Autodesk Inventor part; units mm, degrees
ref_plane "ANBAU_XY" through (0, 5.2, 8.6) normal (0, 0, -1) x (1, 0, 0)
ref_plane "ANBAU_YZ" through (0, 5.2, 8.6) normal (1, 0, 0) x (0, -1, 0)
ref_plane "ANBAU_ZX" through (0, 5.2, 8.6) normal (0, -1, 0) x (0, 0, -1)
sketch "Skizze_1" plane through (0, 0, 0) normal (0, 0, 1) x (1, 0, 0)
  line L0 (-6, 20.5) -> (-6, 0)
  line L1 (-6, 0) -> (6, 0)
  line L2 (6, 0) -> (6, 20.5)
  arc A0 (6, 20.5) -> (2, 24.5) centre (2, 20.5) ccw
  line L3 (2, 24.5) -> (-2, 24.5)
  arc A1 (-2, 24.5) -> (-6, 20.5) centre (-2, 20.5) ccw
extrude "Extrusion1" add sketch "Skizze_1" along normal blind 19
sketch "Skizze_2" plane through (0, 0, 0) normal (1, 0, 0) x (0, 1, 0)
  line L0 (1.5, 8.6) -> (0, 8.6)
  line L1 (0, 8.6) -> (0, 7.734)
  line L2 (0, 7.734) -> (1.5, 8.6)
extrude "Extrusion2" cut sketch "Skizze_2" along normal mid plane 12
sketch "Skizze_5" plane through (0, 0, 0) normal (1, 0, 0) x (0, 1, 0)
  line L0 (5.2, 0) -> (5.2, 8.6)
  line L1 (5.2, 0.6) -> (8.3, 0.6)
  line L2 (8.3, 0.6) -> (8.7, 1)
  line L3 (8.7, 1) -> (8.7, 4.6)
  line L4 (8.7, 4.6) -> (9.2, 4.6)
  line L5 (9.2, 4.6) -> (9.2, 0)
  line L6 (9.2, 0) -> (5.2, 0)
  line L7 (5.2, 0) -> (5.2, 0.6)
sketch "Sketch_1" plane through (0, 0, 8.6) normal (0, 0, 1) x (1, 0, 0)
  line L0 (-6, 24.5) -> (-6, 0)
  line L1 (-6, 0) -> (8, 0)
  line L2 (8, 0) -> (8, 15)
  line L3 (8, 15) -> (6, 15)
  arc A0 (2, 11) -> (6, 15) centre (2, 15) ccw
  line L4 (2, 11) -> (-2.8, 11)
  line L5 (-2.8, 11) -> (-2.8, 24.5)
  line L6 (-2.8, 24.5) -> (-6, 24.5)
extrude "Extrusion3" cut sketch "Sketch_1" along normal blind 19.8
revolve "Revolution1" cut sketch "Skizze_5" angle 360 about axis through (0, 5.2, 0) along (0, 0, -1)
sketch "Skizze_6" plane through (0, 5.2, 0.6) normal (0, 0, -1) x (0, 1, 0)
  line L0 (-1.5, -0.866) -> (0, -1.7321)
  line L1 (0, -1.7321) -> (1.5, -0.866)
  line L2 (1.5, -0.866) -> (1.5, 0.866)
  line L3 (1.5, 0.866) -> (0, 1.7321)
  line L4 (0, 1.7321) -> (-1.5, 0.866)
  line L5 (-1.5, 0.866) -> (-1.5, -0.866)
extrude "Extrusion4" cut sketch "Skizze_6" against normal blind 2
sketch "Skizze_9" plane through (0, 0, 6.45) normal (0, 0, 1) x (1, 0, 0)
  line L0 (-6, 13.5) -> (-5.2, 13.5)
  arc A0 (-5.2, 13.5) -> (-2.8, 15.9) centre (-5.2, 15.9) ccw
  line L1 (-2.8, 15.9) -> (-2.8, 24.5)
  line L2 (-2.8, 24.5) -> (-6, 24.5)
  line L3 (-6, 24.5) -> (-6, 13.5)
extrude "Extrusion5" cut sketch "Skizze_9" along normal mid plane 12.9
sketch "Skizze_13" plane through (0, 0, 0) normal (1, 0, 0) x (0, 1, 0)
  line L0 (10.9, 10.9196) -> (10.9, 8.6)
  line L1 (10.9, 8.6) -> (11.2, 8.6)
  arc A0 (11.2, 8.6) -> (11.7196, 9.5) centre (11.2, 9.2) ccw
  line L2 (11.7196, 9.5) -> (10.9, 10.9196)
extrude "Extrusion6" cut sketch "Skizze_13" along normal mid plane 12
sketch "Sketch_3" plane through (0, 0, 0) normal (0, 1, 0) x (-1, 0, 0)
  line L0 (-2.0163, 19) -> (-6, 19)
  line L1 (-6, 19) -> (-6, 16.7)
  line L2 (-6, 16.7) -> (-2.0163, 19)
extrude "Extrusion7" cut sketch "Sketch_3" along normal mid plane 49
sketch "Sketch_5" plane through (0, 0, 0) normal (1, 0, 0) x (0, 1, 0)
  line L0 (5.2, 8.6) -> (5.2, 12.6)
  line L1 (5.2, 12.6) -> (6.7705, 12.6)
  line L2 (6.7705, 12.6) -> (7.2, 12.1705)
  line L3 (7.2, 12.1705) -> (7.2, 8.6)
  line L4 (7.2, 8.6) -> (5.2, 8.6)
  line L5 (5.2, 8.6) -> (5.2, 12.6)
revolve "Revolution2" add sketch "Sketch_5" angle 360 about axis through (0, 5.2, 8.6) along (0, 0, -1)
thread "Thread1"
ref_plane "ANBAU_XY" through (0, 5.2, 8.6) normal (0, 0, -1) x (1, 0, 0)
ref_plane "ANBAU_YZ" through (0, 5.2, 8.6) normal (1, 0, 0) x (0, -1, 0)
ref_plane "ANBAU_ZX" through (0, 5.2, 8.6) normal (0, -1, 0) x (0, 0, -1)
properties part number "686786 DGSL-12-AS"
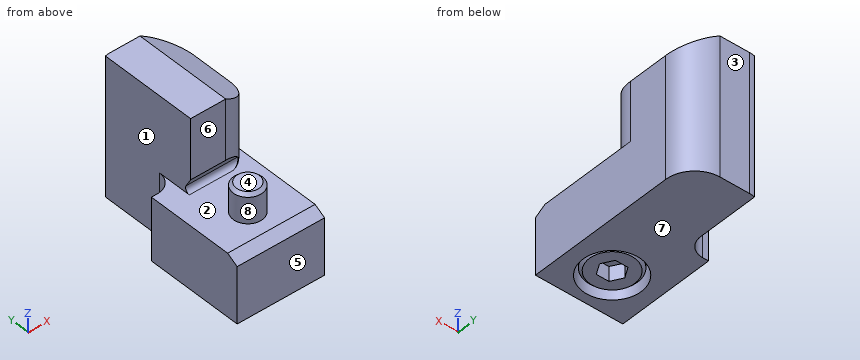
CAD build for the part. Positions are in the model's coordinates, mm. Face numbers are marked on the shaded views. A direction names the side the tool comes from. Coordinates: 2 decimals unless noted, no trailing zeros. Loops run counter-clockwise (first coordinate to the right, second up) from the corner with the lowest first, then second, coordinate; pieces in that order, holes last. Notation, with made-up numbers: (45.5, -16.75) -> (82.5, -16.75) arc R21 ccw to (82.5, 15.25) -> close; hole circle Ø4 at (-10, 81). An arc over 180 degrees is marked (long way). One line per item, written item: value.
1. Slice it at A-A on z = 11.75. Write the cut outline in (x, y), and give its area (3 significant figures).
Answers:
outline: (-2.8, 11) -> (2, 11) arc R4 ccw to (6, 15) -> (6, 20.5) arc R4 ccw to (2, 24.5) -> (-2, 24.5) arc R4 ccw to (-2.8, 24.42) -> close; circle Ø4 at (0, 5.2)
area: 124 mm^2
2. Slice it at D-D on y = 13. Write the cut outline in (x, z), and give its area (3 significant figures).
Answers:
outline: (-6, 0) -> (6, 0) -> (6, 8.6) -> (5.46, 8.6) -> (5.46, 17.01) -> (2.02, 19) -> (-2.8, 19) -> (-2.8, 8.6) -> (-6, 8.6) -> close
area: 186 mm^2
3. Slice it at B-B on z = 6.25. Write the cut outline in (x, y).
Answers:
outline: (-6, 0) -> (6, 0) -> (6, 20.5) arc R4 ccw to (2, 24.5) -> (-2, 24.5) arc R4 ccw to (-2.8, 24.42) -> (-2.8, 15.9) arc R2.4 cw to (-5.2, 13.5) -> (-6, 13.5) -> close
4. Pull direction Y, two halves, no side cores. Call the marked faces 1, 2 and 3: pulls with the +Y half, pulls with the -Y half, needs draft (parallel to the pull), parting line crosses it, or undercut.
Answers:
face 1: needs draft
face 2: undercut
face 3: pulls with the +Y half
5. Drill centre lines: line 1 (Z direction, x = 5, y = 3); line 2 (Z direction, x = 1, y = 2.5); line 3 (X direction, y = 4.5, z = 2). Where is each one in solid material? Low to high. Write a range as [from, to].
Answers:
line 1: z = [0, 8.6]
line 2: z = [0.6, 8.6]
line 3: x = [-6, -3.94], [-3.43, -1.33], [1.33, 3.43], [3.94, 6]
6. Flat gauge pins, fed straight in: P1, Ø0.6, axis at x = -5.5, z = 3.5, coming from the +Y side; P2, Ø1.6, axis at x = 0, y = 5, coming from the +Z side; P3, Ø2.5, axis at x = 0.5, y = 4, coming from the -Z side. Where does each tip first touch, or does it go through?
Answers:
P1: stops at y = 13.5
P2: stops at z = 12.6
P3: stops at z = 0.6
7. Which spindle directions (+Z, -Z, +X, -X, +Y, -Y) get a long thin tool onto all of the face, cutting with end or side? Do the marked faces 4, 5, 6, 7 and 8. Say none if no direction does.
Answers:
face 4: +Z, +X, -X, -Y
face 5: +Z, -Z, +X, -X, -Y
face 6: +Z, +X, -X
face 7: -Z, +X, -X, +Y, -Y
face 8: +Z
